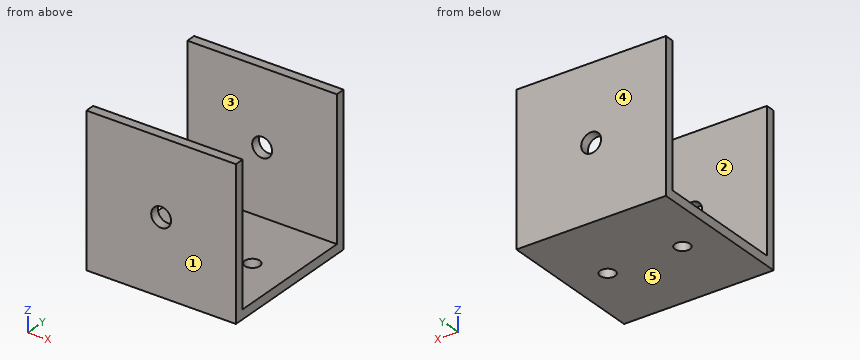
from build123d import *

# Parameters (mm, degrees)
F1_DEPTH = 25.4
F3_D     = 5.1054
F5_D     = 6.7564


with BuildPart() as f1:
    # F0 (on Right) → F1 (new body, symmetric)
    with BuildSketch(Plane.YZ):
        Polygon((-25.4, 50.8), (-25.4, 0), (0, 0), (0, 3.175), (-22.225, 3.175), (-22.225, 50.8), align=None)
        Polygon((0, 3.175), (0, 0), (25.4, 0), (25.4, 50.8), (22.225, 50.8), (22.225, 3.175), align=None)
    extrude(amount=F1_DEPTH, both=True)

    # F3 (through all)
    with Locations(Plane.XY.offset(3.175)):
        with Locations((-12.7, 0), (12.7, 0)):
            Hole(F3_D / 2)

    # F5 (through all)
    with Locations(Plane.XZ.offset(25.4)):
        with Locations((0, 25.4)):
            Hole(F5_D / 2)


solid = f1.part
Could you check a few things on this model? Use its own coordinates, in mm. Face numbers are marked on the shaded views. A direction names the side the tool comes from. Coordinates: 2 decimals unless noted, no trailing zeros. Order: outer loops, then holes, each group sorted by start corner. A loop starts at its lowest first (then second) coordinate and runs counter-clockwise, first axis right, second up. Notation, with made-up numbers: (-4, 71) - (35, 71) arc R24 cw to (35, 93) - close; hole circle Ø10 at (79.25, 31.25). An arc over 180 degrees is marked (long way). Answer in a Markdown table with one row per item. Add a question column.
(1) On a 3-axis mill with a long thin cutter (end or side, diameter ignored), from which of +Z, -Z, +X, -X, +Y, -Y can I reach the whole of each face in a straight line? I mean the marked faces 1 and 2. Say none if no direction works.
(2) If we section it at B-B, the plane z = 25.4: Please give me the cut outline in (x, y) (3 decimals).
(3) If we section it at C-C, the plane x = 0: Please give me the cut outline in (y, z) (3 decimals), then the cut area to 3 significant figures.
(4) If we mould it in two halves opening along Y, with no side actions, what happens to the marked faces 3, 4 and 5? For each: released by +Y, released by -Y, zero draft, split by the parting line, or undercut.
(5) Will this pin go through, and if not, where does the flat tip stop? pin 1 (6 mm diameter, centred on x = -12.7, y = 0, fed in from +Z) (3 decimals).
(6) I need wall thicknesses on L1, parallel to Y at x = -17.5, z = 36 (3 decimals); L2, parallel to Z at x = 0, y = 23.9; L3, parallel to Z at x = -3.5, y = 7 (3 decimals). Which ranges of each line are inside material? Lowest first, please.
(7) If we section it at D-D, the plane y = -7: Please give me the cut outline in (x, z) (3 decimals), then the cut area to 3 significant figures.
(8) If we section it at A-A, the plane x = -12.7: Please give me the cut outline in (y, z) (3 decimals), then the cut area to 4 significant figures.
Results are:
| question | item | result |
|---|---|---|
| 1 | face 1 | +Z, -Z, +X, -X, -Y |
| 1 | face 2 | +Z, +X, -X |
| 2 | outline | (-25.4, -25.4) - (-3.378, -25.4) - (-3.378, -22.225) - (-25.4, -22.225) - close; (-25.4, 22.225) - (-3.378, 22.225) - (-3.378, 25.4) - (-25.4, 25.4) - close; (3.378, -25.4) - (25.4, -25.4) - (25.4, -22.225) - (3.378, -22.225) - close; (3.378, 22.225) - (25.4, 22.225) - (25.4, 25.4) - (3.378, 25.4) - close |
| 3 | outline | (-25.4, 0) - (25.4, 0) - (25.4, 22.022) - (22.225, 22.022) - (22.225, 3.175) - (-22.225, 3.175) - (-22.225, 22.022) - (-25.4, 22.022) - close; (-25.4, 28.778) - (-22.225, 28.778) - (-22.225, 50.8) - (-25.4, 50.8) - close; (22.225, 28.778) - (25.4, 28.778) - (25.4, 50.8) - (22.225, 50.8) - close |
| 3 | area | 421 mm2 |
| 4 | face 3 | undercut |
| 4 | face 4 | released by +Y |
| 4 | face 5 | zero draft |
| 5 | pin 1 | stops at z = 3.175 |
| 6 | L1 | y = -25.4 to -22.225, 22.225 to 25.4 |
| 6 | L2 | z = 0 to 22.02, 28.78 to 50.8 |
| 6 | L3 | z = 0 to 3.175 |
| 7 | outline | (-25.4, 0) - (25.4, 0) - (25.4, 3.175) - (-25.4, 3.175) - close |
| 7 | area | 161 mm2 |
| 8 | outline | (-25.4, 0) - (-2.553, 0) - (-2.553, 3.175) - (-22.225, 3.175) - (-22.225, 50.8) - (-25.4, 50.8) - close; (2.553, 0) - (25.4, 0) - (25.4, 50.8) - (22.225, 50.8) - (22.225, 3.175) - (2.553, 3.175) - close |
| 8 | area | 447.5 mm2 |
